Part model, mm, in its own coordinate system. A direction names the side the tool comes from. Coordinates: 2 decimals unless noted, no trailing zeros. Loops run counter-clockwise (first coordinate to the right, second up) from the corner with the lowest first, then second, coordinate; pieces in that order, holes last. Notation, with made-up numbers: (-27, 24.25) -> (-6, 24.25) arc R23 cw to (-6, 41.25) -> close; hole circle Ø8 at (60.25, -14.75). An arc over 180 degrees is marked (long way). One line per item, written item: value. Start each with the question number.
from build123d import *

# Parameters (mm, degrees)
BOSS_EXTRUDE2_DEPTH = 4
CUT_EXTRUDE3_DEPTH  = 4
SKETCH6_R           = 46.644893749
CUT_EXTRUDE4_DEPTH  = 2
SKETCH7_W           = 37.921763703
SKETCH7_H           = 21.966033547
CUT_EXTRUDE5_DEPTH  = 2
CUT_EXTRUDE7_DEPTH  = 10
BOSS_EXTRUDE3_DEPTH = 2


with BuildPart() as part:
    # Sketch4 → Boss-Extrude2 (new body)
    with BuildSketch(Plane(origin=(0, 0, 0), x_dir=(1, 0, 0), z_dir=(0, 1, 0))):
        with BuildLine():
            Line((-107.035735829, 49.14195745), (-15.035735829, 49.14195745))
            Line((-15.035735829, 49.14195745), (-15.035735829, -45.85804255))
            ThreePointArc((-15.035735829, -45.85804255), (-16.500201924, -49.393576456), (-20.035735829, -50.85804255))
            Line((-20.035735829, -50.85804255), (-102.035735829, -50.85804255))
            ThreePointArc((-102.035735829, -50.85804255), (-105.571269735, -49.393576456), (-107.035735829, -45.85804255))
            Line((-107.035735829, -45.85804255), (-107.035735829, 49.14195745))
        make_face()
    extrude(amount=BOSS_EXTRUDE2_DEPTH)

    # Sketch5 → Cut-Extrude3 (cut)
    with BuildSketch(Plane(origin=(0, 4, 0), x_dir=(1, 0, 0), z_dir=(0, 1, 0))):
        with BuildLine():
            Line((-122.184107688, 54.312207558), (-0.881081782, 54.312207558))
            Line((-0.881081782, 54.312207558), (-0.881081782, -1.763818638))
            Line((-0.881081782, -1.763818638), (-15.035735829, -1.763818638))
            ThreePointArc((-15.035735829, -1.763818638), (-61.035735829, 48.088703252), (-107.035735829, -1.763818638))
            Line((-107.035735829, -1.763818638), (-116.20594022, -1.763818638))
            Line((-116.20594022, -1.763818638), (-122.184107688, 54.312207558))
        make_face()
    extrude(amount=-CUT_EXTRUDE3_DEPTH, mode=Mode.SUBTRACT)

    # Sketch6 → Cut-Extrude4 (cut)
    with BuildSketch(Plane(origin=(0, 4, 0), x_dir=(1, 0, 0), z_dir=(0, 1, 0))):
        with Locations((-61.039241489, 3.84195745)):
            Circle(SKETCH6_R)
    extrude(amount=-CUT_EXTRUDE4_DEPTH, mode=Mode.SUBTRACT)

    # Sketch7 → Cut-Extrude5 (cut)
    with BuildSketch(Plane(origin=(0, 2, 0), x_dir=(1, 0, 0), z_dir=(0, 1, 0))):
        with Locations((-69.228954178, 3.760987583)):
            Rectangle(SKETCH7_W, SKETCH7_H)
    extrude(amount=-CUT_EXTRUDE5_DEPTH, mode=Mode.SUBTRACT)

    # Sketch13 → Cut-Extrude7 (cut)
    with BuildSketch(Plane(origin=(0, 2, 0), x_dir=(1, 0, 0), z_dir=(0, 1, 0))):
        with BuildLine():
            Line((-106.217317024, -1.560957592), (-107.035735829, -3.908437462))
            Line((-107.035735829, -3.908437462), (-110.118060938, -1.560957592))
            ThreePointArc((-110.118060938, -1.560957592), (-61.039241489, 53.217275266), (-11.960422041, -1.560957592))
            Line((-11.960422041, -1.560957592), (-15.035735829, -3.816260145))
            Line((-15.035735829, -3.816260145), (-15.861165954, -1.560957592))
            ThreePointArc((-15.861165954, -1.560957592), (-61.039241489, 49.34195745), (-106.217317024, -1.560957592))
        make_face()
    extrude(amount=-CUT_EXTRUDE7_DEPTH, mode=Mode.SUBTRACT)

    # Sketch10 → Boss-Extrude3 (add)
    with BuildSketch(Plane(origin=(0, 4, 0), x_dir=(1, 0, 0), z_dir=(0, 1, 0))):
        with BuildLine():
            Line((-110.035735829, -0.626443871), (-107.035735829, -0.626443871))
            Line((-107.035735829, -0.626443871), (-107.035735829, -3.908437462))
            ThreePointArc((-107.035735829, -3.908437462), (-97.412251623, -25.359930275), (-78.547707812, -39.392284997))
            Line((-78.547707812, -39.392284997), (-78.547707812, -53.939312876))
            Line((-78.547707812, -53.939312876), (-105.035735829, -53.939312876))
            ThreePointArc((-105.035735829, -53.939312876), (-108.571269735, -52.474846782), (-110.035735829, -48.939312876))
            Line((-110.035735829, -48.939312876), (-110.035735829, -0.626443871))
        make_face()
        with BuildLine():
            Line((-12.035735829, -0.626443871), (-12.035735829, -48.939312876))
            ThreePointArc((-12.035735829, -48.939312876), (-13.500201924, -52.474846782), (-17.035735829, -53.939312876))
            Line((-17.035735829, -53.939312876), (-43.530775166, -53.939312876))
            Line((-43.530775166, -53.939312876), (-43.530775166, -39.392284997))
            ThreePointArc((-43.530775166, -39.392284997), (-24.652990845, -25.343430622), (-15.035735829, -3.86671169))
            Line((-15.035735829, -3.86671169), (-15.035735829, -0.626443871))
            Line((-15.035735829, -0.626443871), (-12.035735829, -0.626443871))
        make_face()
    extrude(amount=BOSS_EXTRUDE3_DEPTH)


solid = part.part
1) Pull direction Z, two halves, no side cores. Call faces 4 (the flat face through (-24, 6, 39)), 5 (the cylindrical face through (-15.78, 1.01, -8.5)), 6 (the cylindrical face through (-16.462, 1.972, 49.354)): +Z half, -Z half, draft (parallel to the pull), parting line (faces both ways), or undercut.
2) Slice it at C-C (x = -63.5). Give the cut face in (y, z).
3) Slice it at D-D (x = -42). Give the cut face in (y, z), then the cut area to 3 significant figures.
4) Slice it at A-A (y = 1.1). Give the cut face in (x, z), then the cut area to 3 significant figures.
5) Slice it at B-B (z = -1). Give the cut face in (x, y).
6) Probe line 1 (X direction, y = 5.3, z = 1); line 2 (Z direction, x = -61.5, y = 0.3); line 3 (X direction, y = 5.35, z = 7.5). List the from-to ranges inside material, lowest first. Write a range as from..to.
7) Pin check, flat tips, straight feed: pin 1 Ø3 at (x, y) = (-43.5, 2) entering from -Z; pin 2 Ø1.5 at (x, y) = (-82.5, 1.5) entering from +Z; pin 3 Ø1.5 at (x, z) = (-96, -27) entering from +Y; pin 4 Ø15.5 at (x, z) = (-98, 19.5) entering from -Y. Stop position of each tip, or through.
8) Tool access for faces 1 (the flat face through (-60, 2, 50.858)), 2 (the flat face through (-107.036, 2, 25)), 3 (the flat face through (-108, 4, 33)): list every direction of +Z, -Z, +X, -X, +Y, -Y with a clear straight run to the whole face (end or side of a thin tool).
Check sheet entries:
1. face 4: draft
1. face 5: undercut
1. face 6: +Z half
2. outline: (0, -48.02) -> (2, -48.02) -> (2, -14.74) -> (0, -14.74) -> close; (0, 7.22) -> (2, 7.22) -> (2, 42.74) -> (4, 42.74) -> (4, 50.86) -> (0, 50.86) -> close
3. outline: (0, -43.98) -> (2, -43.98) -> (2, 38.74) -> (6, 38.74) -> (6, 53.94) -> (4, 53.94) -> (4, 50.86) -> (0, 50.86) -> close
3. area: 244 mm^2
4. outline: (-107.04, 3.91) -> (-106.22, 1.56) arc R45.5 ccw to (-104.13, -18.44) arc R46.15 ccw to (-18, -18.6) arc R45.5 ccw to (-15.86, 1.56) -> (-15.04, 3.82) -> (-15.04, 45.86) arc R5 ccw to (-20.04, 50.86) -> (-102.04, 50.86) arc R5 ccw to (-107.04, 45.86) -> close; hole (-88.19, -14.74) -> (-50.27, -14.74) -> (-50.27, 7.22) -> (-88.19, 7.22) -> close
4. area: 7,340 mm^2
5. outline: (-106.45, 0) -> (-88.19, 0) -> (-88.19, 2) -> (-106.45, 2) -> close; (-50.27, 0) -> (-15.63, 0) -> (-15.63, 2) -> (-50.27, 2) -> close
6. line 1: x = -110.04..-107.04, -15.04..-12.04
6. line 2: z = -48.09..-14.74, 7.22..50.86
6. line 3: x = -110.04..-106.28, -15.79..-12.04
7. pin 1: stops at z = -45.21
7. pin 2: stops at z = 50.86
7. pin 3: stops at y = 2
7. pin 4: stops at y = 0
8. face 1: +Z, +X, -X, -Y
8. face 2: +Z, -Z, -X, -Y
8. face 3: +Z, -X, -Y
